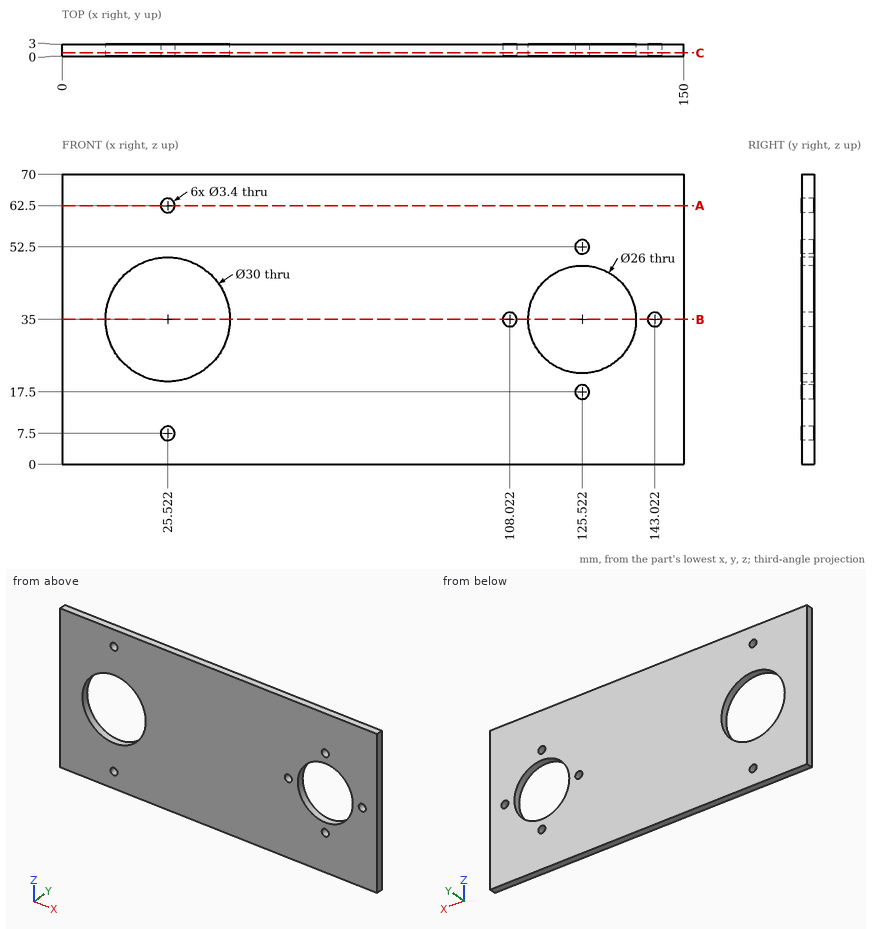
Answer from the drawing. Dimensions are ordinates in mm from the lowest x, y and z of the part. Round coordinates to 2 decimals unless told otherwise and drop trailing zeros. Order: outer loops, then holes, each group sorted by start corner. A loop starts at its lowest first (then second) coordinate and runs counter-clockwise, first axis right, second up.
1) The part is cut by section A-A on z = 62.5. Write down the section's boundary in (x, y).
2) The part is cut by section C-C on y = 0.85. Give the number of separate pieces and of enclosed holes in the cut face, plus the area to 3 significant figures.
3) A flat-ended cylindrical pin translates along its axis: pin 1 (5.5 mm diameter, centred on x = 25.52, z = 62.5, fed in from +Y). Find the tip coordinate at first contact, or state that the pin passes through.
4) The part is cut by section B-B on z = 35. Write down the section's boundary in (x, y).
5) Straight lines are drawn through the part: L1, parallel to X at y = 1.35, z = 35; L2, parallel to Z at x = 18, y = 2.85; L3, parallel to X at y = 1.1, z = 7.5. For each, find the intervals that lie inside material, in ascending order.
Resolved:
1. outline: (0, 0) - (23.82, 0) - (23.82, 3) - (0, 3) - close; (27.22, 0) - (150, 0) - (150, 3) - (27.22, 3) - close
2. separate pieces: 1
2. enclosed holes: 8
2. area: 9,210 mm2
3. pin 1: stops at y = 3
4. outline: (0, 0) - (10.52, 0) - (10.52, 3) - (0, 3) - close; (40.52, 0) - (106.32, 0) - (106.32, 3) - (40.52, 3) - close; (109.72, 0) - (112.52, 0) - (112.52, 3) - (109.72, 3) - close; (138.52, 0) - (141.32, 0) - (141.32, 3) - (138.52, 3) - close; (144.72, 0) - (150, 0) - (150, 3) - (144.72, 3) - close
5. L1: x = 0 to 10.52, 40.52 to 106.32, 109.72 to 112.52, 138.52 to 141.32, 144.72 to 150
5. L2: z = 0 to 22.02, 47.98 to 70
5. L3: x = 0 to 23.82, 27.22 to 150
